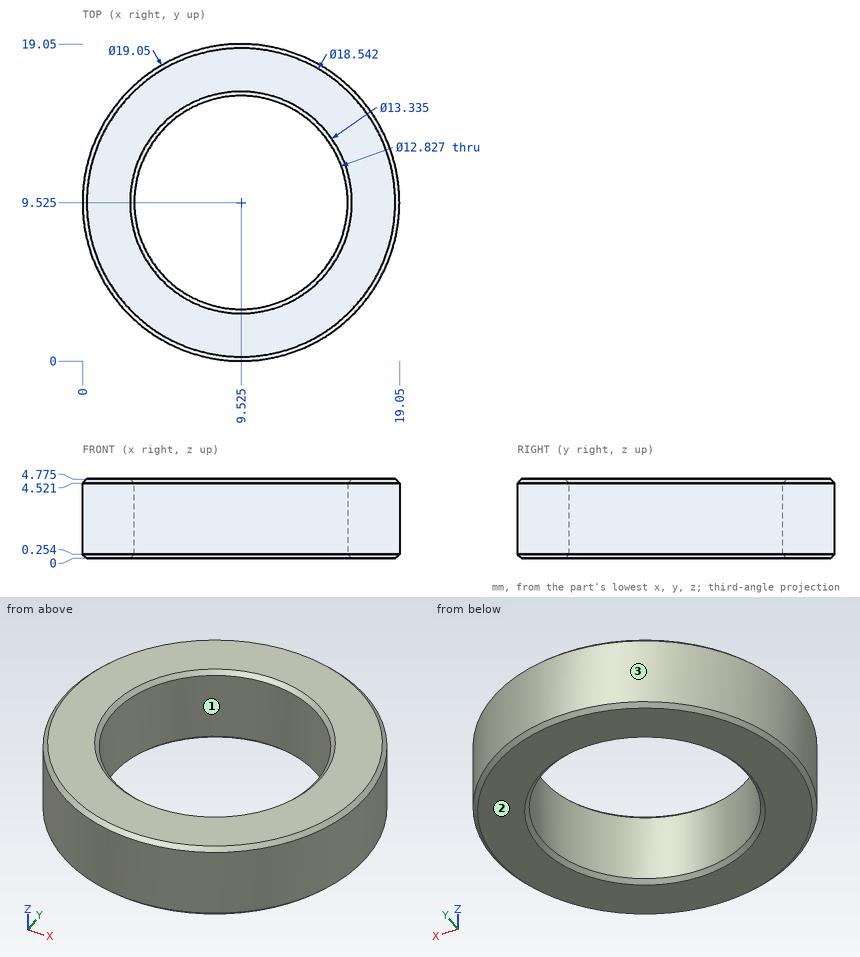
Can you work these out from the drawing? Everything is in mm from the part's minimum corner. Coordinates: 2 decimals unless noted, no trailing zeros. Return JSON: item names as keys, results as strings.
1) I need wall thicknesses on line 1 (X direction, y = 9.5, z = 0.3); line 2 (Y direction, x = 9.75, z = 1.65); line 3 (Y direction, x = 5.25, z = 2.8) (1 decimal). Which ranges of each line are inside material? Lowest first, please. Write a range as from..to.
Results below:
{"line 1": "0..3.11, 15.94..19.05", "line 2": "0..3.12, 15.93..19.05", "line 3": "1..4.7, 14.3..18"}
2) Thinking about a two-plate mould opening in X: for the marked faces 1, 2 and 3, which applies, +X half, -X half, draft (parallel to the pull), parting line (faces both ways), or undercut?
Results below:
{"face 1": "undercut", "face 2": "draft", "face 3": "parting line"}
3) Will this pin go through, and if not, where does the flat tip stop? pin 1 (1 mm diameter, centred on x = 7.5, y = 15, fed in from -Z).
Results below:
{"pin 1": "through"}
